Check sheet for the modelled part. Datum: model origin and axes. Units: mm. A direction names the side the tool comes from. Give positions to 0.01 mm unless a question says otherwise; leave off trailing zeros. Order: outer loops, then holes, each group sorted by start corner. A loop starts at its lowest first (then second) coordinate and runs counter-clockwise, first axis right, second up. Notation, with made-up numbers: (33.5, -39.75) -> (88.5, -39.75) arc R21 ccw to (88.5, -3.75) -> close; hole circle Ø4 at (-26.5, 11.25). An arc over 180 degrees is marked (long way). Answer in a Markdown table with one row per item. Add a question column.
(1) Cross-section at B-B (x = 7.5). Record the cut outline in (y, z).
(2) Go/stop test with flat-tipped pins: pin 1 (1.5 mm diameter, centred on y = 8, z = 1, fed in from -X); pin 2 (6.5 mm diameter, centred on x = -38.89, y = 38.89, fed in from +Z); pin 3 (1.5 mm diameter, centred on x = 27.5, z = 1.5, fed in from +Y). Record where each tip stops, or that it passes through.
(3) Cross-section at A-A (z = 1.05). Record the cut outline in (x, y), then the cut area to 3 significant figures.
(4) Set-up check for faces 1 (the face through (33, 5, 1)), 2 (the face through (32, -5, 1)): record each of +Z, -Z, +X, -X, +Y, -Y from which the full face is reachable in a straight line by a thin tool's end or side.
(5) Cross-section at C-C (y = 33). Record the cut outline in (x, z).
(6) Thickness scan on L1, parallel to Y at x = 21, z = 0.4; L2, parallel to Y at x = -37.5, z = 2.3; L3, parallel to Y at x = -37, z = 2.4. Record the ranges inside material, lowest first. Write a range as [from, to].
```python
from build123d import *

# Parameters (mm, degrees)
BOSS_EXTRUDE1_DEPTH = 3
SKETCH3_R           = 2.5
CUT_EXTRUDE1_DEPTH  = 11


with BuildPart() as part:
    # Sketch2 → Boss-Extrude1 (new body)
    with BuildSketch(Plane.XY):
        with BuildLine():
            Line((2.071067812, 5), (65, 5))
            ThreePointArc((65, 5), (70, 0), (65, -5))
            Line((65, -5), (-2.071067812, -5))
            Line((-2.071067812, -5), (-42.426406871, 35.355339059))
            ThreePointArc((-42.426406871, 35.355339059), (-42.426406871, 42.426406871), (-35.355339059, 42.426406871))
            Line((-35.355339059, 42.426406871), (2.071067812, 5))
        make_face()
    extrude(amount=BOSS_EXTRUDE1_DEPTH)

    # Sketch3 → Cut-Extrude1 (cut)
    with BuildSketch(Plane.XY.offset(3)):
        with Locations((-38.890872965, 38.890872965)):
            Circle(SKETCH3_R)
    extrude(amount=-CUT_EXTRUDE1_DEPTH, mode=Mode.SUBTRACT)


solid = part.part
```
Answer below:
| question | item | result |
|---|---|---|
| 1 | outline | (-5, 0) -> (5, 0) -> (5, 3) -> (-5, 3) -> close |
| 2 | pin 1 | stops at x = -15.82 |
| 2 | pin 2 | stops at z = 3 |
| 2 | pin 3 | stops at y = 5 |
| 3 | outline | (-42.43, 35.36) -> (-2.07, -5) -> (65, -5) arc R5 ccw to (65, 5) -> (2.07, 5) -> (-35.36, 42.43) arc R5 ccw to start; hole circle Ø5 at (-38.89, 38.89) |
| 3 | area | 1,260 mm² |
| 4 | face 1 | +Z, -Z, +X, +Y |
| 4 | face 2 | +Z, -Z, +X, -X, -Y |
| 5 | outline | (-40.07, 0) -> (-25.93, 0) -> (-25.93, 3) -> (-40.07, 3) -> close |
| 6 | L1 | y = [-5, 5] |
| 6 | L2 | y = [30.43, 36.81], [40.97, 43.69] |
| 6 | L3 | y = [29.93, 37.26], [40.53, 43.52] |
